from build123d import *

# Parameters (mm, degrees)
BOSS_EXTRUDE1_DEPTH  = 11.45
M6_CLEARANCE_HOLE1_D = 6.4
FILLET1_R            = 1


with BuildPart() as part:
    # Sketch1 → Boss-Extrude1 (new body)
    with BuildSketch(Plane(origin=(0, 0, 0), x_dir=(1, 0, 0), z_dir=(0, 1, 0))):
        with BuildLine():
            Line((13.919410907, 37.5), (-13.919410907, 37.5))
            ThreePointArc((-13.919410907, 37.5), (-28.284271247, 28.284271247), (-37.5, 13.919410907))
            Line((-37.5, 13.919410907), (-37.5, -13.919410907))
            ThreePointArc((-37.5, -13.919410907), (-28.284271247, -28.284271247), (-13.919410907, -37.5))
            Line((-13.919410907, -37.5), (13.919410907, -37.5))
            ThreePointArc((13.919410907, -37.5), (28.284271247, -28.284271247), (37.5, -13.919410907))
            Line((37.5, -13.919410907), (37.5, 13.919410907))
            ThreePointArc((37.5, 13.919410907), (28.284271247, 28.284271247), (13.919410907, 37.5))
        make_face()
        with BuildLine():
            ThreePointArc((22.5, 0), (-13.205112646, -18.217436702), (-7, 21.38340478))
            Line((-7, 21.38340478), (-7, 27.38340478))
            Line((-7, 27.38340478), (7, 27.38340478))
            Line((7, 27.38340478), (7, 21.38340478))
            ThreePointArc((7, 21.38340478), (18.217436702, 13.205112646), (22.5, 0))
        make_face(mode=Mode.SUBTRACT)
    extrude(amount=-BOSS_EXTRUDE1_DEPTH)

    # M6 Clearance Hole1 (through all)
    with Locations(Plane(origin=(-30, 0, 0), x_dir=(0, 0, 1), z_dir=(0, 1, 0))):
        with Locations((0, 0), (-25.980762114, 15), (-25.980762114, 45), (0, 60), (25.980762114, 45), (25.980762114, 15)):
            Hole(M6_CLEARANCE_HOLE1_D / 2)

    # Fillet1
    fillet1_edges = [part.edges().sort_by_distance(p)[0] for p in [
        (7, -5.725, -21.38340478),
        (7, -5.725, -27.38340478),
        (-7, -5.725, -27.38340478),
        (-7, -5.725, -21.38340478),
    ]]
    fillet(fillet1_edges, radius=FILLET1_R)


solid = part.part
For this review, take the finished solid that the model builds, in its own axes (mm). A direction names the side the tool comes from. Round coordinates to 2 decimals unless told otherwise and drop trailing zeros. Write each loop counter-clockwise with the first axis right and the second up, starting at its lowest first coordinate (ties: lowest second). Pieces come first, ordered by that corner, then holes. Notation, with made-up numbers: (84, 74.25) -> (128, 74.25) arc R29 cw to (128, 107.25) -> close; hole circle Ø9 at (73, 86). An arc over 180 degrees is marked (long way). Put each result on its own line as item: value.
Q1. Machinability: for faces 1 (the flat face through (7, -6, -24)), 2 (the flat face through (-17, -11.45, 16)), which of the approach directions +Z, -Z, +X, -X, +Y, -Y give a long, thin tool a straight path to every point of the face, cutting with its end or side? Answer none if there is none.
Determined:
face 1: +Y, -Y
face 2: +Z, -Z, +X, -X, -Y
Q2. Consider section B-B on y = -2.5. State the section outline as (x, z) points, and give its area (3 significant figures).
Determined:
outline: (-37.5, -13.92) arc R40 ccw to (-13.92, -37.5) -> (13.92, -37.5) arc R40 ccw to (37.5, -13.92) -> (37.5, 13.92) arc R40 ccw to (13.92, 37.5) -> (-13.92, 37.5) arc R40 ccw to (-37.5, 13.92) -> close; hole circle Ø6.4 at (-30, 0); hole circle Ø6.4 at (-15, -25.98); hole circle Ø6.4 at (-15, 25.98); hole (-7.66, -21.16) arc R1 cw to (-7, -22.1) -> (-7, -26.38) arc R1 ccw to (-6, -27.38) -> (6, -27.38) arc R1 ccw to (7, -26.38) -> (7, -22.1) arc R1 cw to (7.66, -21.16) arc R22.5 ccw (long way) to start; hole circle Ø6.4 at (15, -25.98); hole circle Ø6.4 at (15, 25.98); hole circle Ø6.4 at (30, 0)
area: 2,980 mm^2
Q3. To check wall thickness, follow L1, parallel to X at y = -1, z = 0; L2, parallel to X at y = -4, z = 27; L3, parallel to X at y = -4, z = -7. State the ranges of each line that lie inside material, in increasing order. Write a range as [from, to].
Determined:
L1: x = [-37.5, -33.2], [-26.8, -22.5], [22.5, 26.8], [33.2, 37.5]
L2: x = [-29.51, -18.03], [-11.97, 11.97], [18.03, 29.51]
L3: x = [-37.5, -21.38], [21.38, 37.5]
Q4. Consider section C-C on z = 21. State the section outline as (x, y) points.
Determined:
outline: (-34.04, -11.45) -> (-8.08, -11.45) -> (-8.08, 0) -> (-34.04, 0) -> close; (8.08, -11.45) -> (34.04, -11.45) -> (34.04, 0) -> (8.08, 0) -> close
Q5. The part is to be moulded in two halves that separate along Z. For faces 3 (the cylindrical face through (12.161, -5.805, 24.504)), 4 (the flat face through (0, -6, -37.5)), 5 (the flat face through (0, -6, -27.383)), 6 (the cylindrical face through (28.113, -5.645, 28.454)), say which applies: released by +Z, released by -Z, zero draft, split by the parting line, or undercut.
Determined:
face 3: undercut
face 4: released by -Z
face 5: undercut
face 6: released by +Z
Q6. Consider section A-A on x = 0. State the section outline as (y, z) points, and give its area (3 significant figures).
Determined:
outline: (-11.45, -37.5) -> (0, -37.5) -> (0, -27.38) -> (-11.45, -27.38) -> close; (-11.45, 22.5) -> (0, 22.5) -> (0, 37.5) -> (-11.45, 37.5) -> close
area: 288 mm^2
Q7. Consider section D-D on x = 15. State the section outline as (y, z) points, and give its area (3 significant figures).
Determined:
outline: (-11.45, -37.08) -> (0, -37.08) -> (0, -29.18) -> (-11.45, -29.18) -> close; (-11.45, -22.78) -> (0, -22.78) -> (0, -16.77) -> (-11.45, -16.77) -> close; (-11.45, 16.77) -> (0, 16.77) -> (0, 22.78) -> (-11.45, 22.78) -> close; (-11.45, 29.18) -> (0, 29.18) -> (0, 37.08) -> (-11.45, 37.08) -> close
area: 319 mm^2
Q8. Clearance check with flat-ended pins moving along their axes: pin 1 Ø1.3 at (y, z) = (-6, -24) entering from -X; pin 2 Ø1 at (x, y) = (19.5, -5.5) entering from +Z; pin 3 Ø1.3 at (y, z) = (-6, -24) entering from +X. State where each tip first meets the part, or that it passes through.
Determined:
pin 1: stops at x = -32.48
pin 2: stops at z = 35.2
pin 3: stops at x = 32.48
